from build123d import *

# Parameters (mm, degrees)
EXTRUDE_START       = -2
EXTRUDE_1_DEPTH     = 2
SKETCH_2_R          = 0.6
SKETCH_2_R_2        = 1.25
EXTRUDE_2_DEPTH     = 2
SKETCH_3_R          = 5.9
SKETCH_3_R_2        = 1.25
EXTRUDE_3_DEPTH     = 18.5
EXTRUDE_4_DEPTH     = 3
SKETCH_5_R          = 1.7
CUT_EXTRUDE_1_DEPTH = 3
SKETCH_6_R          = 1.7
EXTRUDE_5_DEPTH     = 4


# Read off the part's stored shape, not the designer's step: 填料-伸長1
with BuildPart() as part:
    # 填料-伸長1 outline → 填料-伸長1 (new body)
    with BuildSketch(Plane(origin=(0, 18.156954032, 0), x_dir=(1, 0, 0), z_dir=(0, 1, 0)).offset(EXTRUDE_START)):
        with BuildLine():
            Line((-71.976510321, -204.833021781), (-61.351692907, -213.569524655))
            ThreePointArc((-61.351692907, -213.569524655), (-59.430720516, -215.948258819), (-56.577073779, -217.046080048))
            Line((-56.577073779, -217.046080048), (-45.000342303, -224.475246616))
            ThreePointArc((-45.000342303, -224.475246616), (-39.06215434, -223.480955011), (-39.939141491, -217.524312868))
            Line((-39.939141491, -217.524312868), (-50.563958905, -208.787809993))
            ThreePointArc((-50.563958905, -208.787809993), (-52.484931295, -206.409075829), (-55.338578032, -205.311254601))
            Line((-55.338578032, -205.311254601), (-66.915309509, -197.882088033))
            ThreePointArc((-66.915309509, -197.882088033), (-72.853497472, -198.876379638), (-71.976510321, -204.833021781))
        make_face()
        with BuildLine():
            ThreePointArc((-55.939819286, -215.078625755), (-58.253468106, -214.331448143), (-59.674933886, -212.358967399))
            Line((-59.674933886, -212.358967399), (-70.741141252, -203.259521387))
            ThreePointArc((-70.741141252, -203.259521387), (-71.236686796, -200.053632048), (-68.033499603, -199.540910248))
            Line((-68.033499603, -199.540910248), (-55.975832526, -207.278708894))
            ThreePointArc((-55.975832526, -207.278708894), (-53.662183706, -208.025886506), (-52.240717926, -209.998367249))
            Line((-52.240717926, -209.998367249), (-41.17451056, -219.097813262))
            ThreePointArc((-41.17451056, -219.097813262), (-40.678965016, -222.303702601), (-43.882152209, -222.8164244))
            Line((-43.882152209, -222.8164244), (-55.939819286, -215.078625755))
        make_face(mode=Mode.SUBTRACT)
    extrude(amount=EXTRUDE_1_DEPTH)

    # 草圖2 → 填料-伸長2 (add)
    with BuildSketch(Plane(origin=(0, 18.156954032, 0), x_dir=(1, 0, 0), z_dir=(0, 1, 0))):
        with BuildLine():
            Line((-56.577073779, -217.046080048), (-45.000342303, -224.475246616))
            ThreePointArc((-45.000342303, -224.475246616), (-39.06215434, -223.480955011), (-39.939141491, -217.524312868))
            Line((-39.939141491, -217.524312868), (-50.563958905, -208.787809993))
            ThreePointArc((-50.563958905, -208.787809993), (-52.484931296, -206.409075829), (-55.338578032, -205.311254601))
            Line((-55.338578032, -205.311254601), (-66.915309509, -197.882088033))
            ThreePointArc((-66.915309509, -197.882088033), (-72.853497472, -198.876379638), (-71.976510321, -204.833021781))
            Line((-71.976510321, -204.833021781), (-61.351692907, -213.569524655))
            ThreePointArc((-61.351692907, -213.569524655), (-59.430720516, -215.948258819), (-56.577073779, -217.046080048))
        make_face()
        with Locations(Location((-69.943238255, -200.995433976, 0), (0, 0, 180))):
            Circle(SKETCH_2_R, mode=Mode.SUBTRACT)
        with Locations(Location((-68.245587045, -202.231549007, 0), (0, 0, 180))):
            Circle(SKETCH_2_R, mode=Mode.SUBTRACT)
        with Locations(Location((-66.547935835, -203.467664037, 0), (0, 0, 180))):
            Circle(SKETCH_2_R, mode=Mode.SUBTRACT)
        with Locations(Location((-64.850284625, -204.703779068, 0), (0, 0, 180))):
            Circle(SKETCH_2_R, mode=Mode.SUBTRACT)
        with Locations(Location((-63.152633415, -205.939894099, 0), (0, 0, 180))):
            Circle(SKETCH_2_R, mode=Mode.SUBTRACT)
        with Locations(Location((-61.454982205, -207.17600913, 0), (0, 0, 180))):
            Circle(SKETCH_2_R, mode=Mode.SUBTRACT)
        with Locations(Location((-55.957825906, -211.178667324, 0), (0, 0, 180))):
            Circle(SKETCH_2_R_2, mode=Mode.SUBTRACT)
        with Locations(Location((-50.460669607, -215.181325519, 0), (0, 0, 180))):
            Circle(SKETCH_2_R, mode=Mode.SUBTRACT)
        with Locations(Location((-48.763018397, -216.41744055, 0), (0, 0, 180))):
            Circle(SKETCH_2_R, mode=Mode.SUBTRACT)
        with Locations(Location((-47.065367187, -217.65355558, 0), (0, 0, 180))):
            Circle(SKETCH_2_R, mode=Mode.SUBTRACT)
        with Locations(Location((-45.367715977, -218.889670611, 0), (0, 0, 180))):
            Circle(SKETCH_2_R, mode=Mode.SUBTRACT)
        with Locations(Location((-43.670064767, -220.125785642, 0), (0, 0, 180))):
            Circle(SKETCH_2_R, mode=Mode.SUBTRACT)
        with Locations(Location((-41.972413557, -221.361900673, 0), (0, 0, 180))):
            Circle(SKETCH_2_R, mode=Mode.SUBTRACT)
    extrude(amount=EXTRUDE_2_DEPTH)

    # 草圖3 → 填料-伸長3 (add)
    with BuildSketch(Plane(origin=(0, 20.156954032, 0), x_dir=(1, 0, 0), z_dir=(0, 1, 0))):
        with Locations(Location((-55.957825906, -211.178667324, 0), (0, 0, 180))):
            Circle(SKETCH_3_R)
        with Locations(Location((-55.957825906, -211.178667324, 0), (0, 0, 180))):
            Circle(SKETCH_3_R_2, mode=Mode.SUBTRACT)
    extrude(amount=EXTRUDE_3_DEPTH)

    # 草圖4 → 填料-伸長4 (add)
    with BuildSketch(Plane(origin=(0, 38.656954032, 0), x_dir=(1, 0, 0), z_dir=(0, 1, 0))):
        Polygon((-59.623386181, -215.801833758), (-58.127150876, -205.691953447), (-122.426781037, -196.175779785), (-123.923016342, -206.285660097), align=None)
    extrude(amount=-EXTRUDE_4_DEPTH)

    # 草圖5 → 除料-伸長1 (cut)
    with BuildSketch(Plane.XZ.offset(-35.656954032)):
        with Locations((-65.8500767, 209.714640607)):
            Circle(SKETCH_5_R)
    extrude(amount=-CUT_EXTRUDE_1_DEPTH, mode=Mode.SUBTRACT)

    # 草圖6 → 填料-伸長5 (add)
    with BuildSketch(Plane(origin=(0, 28, 0), x_dir=(1, 0, 0), z_dir=(0, 1, 0))):
        with BuildLine():
            Line((-70.340889788, -205.906137252), (-71.251514406, -212.059117246))
            ThreePointArc((-71.251514406, -212.059117246), (-70.879084415, -213.543853469), (-69.565869591, -214.330372748))
            Line((-69.565869591, -214.330372748), (-59.623386181, -215.801833758))
            ThreePointArc((-59.623386181, -215.801833758), (-61.794253874, -210.314891561), (-58.127150876, -205.691953447))
            Line((-58.127150876, -205.691953447), (-68.069634286, -204.220492436))
            ThreePointArc((-68.069634286, -204.220492436), (-69.554370509, -204.592922428), (-70.340889788, -205.906137252))
        make_face()
        with Locations((-65.8500767, -209.714640607)):
            Circle(SKETCH_6_R, mode=Mode.SUBTRACT)
    extrude(amount=EXTRUDE_5_DEPTH)


solid = part.part
Read the model definition and answer for the solid it produces. Units are mm, in the model's axes. A direction names the side the tool comes from. Give positions to 0.01 mm unless a question says otherwise; leave off trailing zeros. Write each loop counter-clockwise with the first axis right and the second up, starting at its lowest first coordinate (ties: lowest second). Pieces come first, ordered by that corner, then holes. Notation, with made-up numbers: M 71,18.25 L 82,18.25 A27 cw 82,51.25 Z; hole C -6,-0.75 d8. An arc over 180 degrees is marked long. One line per item, written item: value. Start each with the question number.
(1) Find section B-B (x = -117.5). Determine the outline of the cut face in (y, z), plus the area to 3 significant figures.
(2) Flat-ended cylindrical pins translate along their axes: pin 1 Ø12 at (y, z) = (31, 210.5) entering from +X; pin 2 Ø1 at (x, z) = (-45.37, 218.89) entering from -Y; pin 3 Ø12 at (x, y) = (-86.5, 33) entering from +Z; pin 4 Ø6 at (x, z) = (-98, 203.5) entering from -Y. Find the tip coordinate at first contact, or state that the pin passes through.
(3) Determine the mould class of faces 4 (the flat face through (-68, 32, 210)), 5 (the cylindrical face through (-69.54, 29.97, 204.58)), 6 (the cylindrical face through (-56.63, 28.263, 212.233)), 7 (the flat face through (-56, 16.157, 207)) for opening direction Y: pulls with the +Y half, pulls with the -Y half, needs draft (parallel to the pull), parting line crosses it, or undercut.
(4) Find section C-C (y = 22). Determine the outline of the cut face in (x, z), plus the area to 3 significant figures.
(5) Find section A-A (y = 30.25). Determine the outline of the cut face in (x, z).
(6) Find the intervals of material crossed by line 1 (Y direction, x = -106.5, z = 201.5); line 2 (Y direction, x = -52.5, z = 218.25); line 3 (X direction, y = 19.75, z = 218.75), in increasing order.
(7) A tool of negligible diameter and unlimited length cuts with its end or side. For faces 1 (the flat face through (-123.164, 37.178, 201.16)), 2 (the cylindrical face through (-66.219, 37.136, 208.055)), 3 (the cylindrical face through (-53.7, 17.1, 208)), from which of +Z, -Z, +X, -X, +Y, -Y can it reach the whole face along a straight path? Write none if from no direction.
Results below:
1. outline: M 35.66,196.9 L 38.66,196.9 L 38.66,207.24 L 35.66,207.24 Z
1. area: 31.0 mm^2
2. pin 1: stops at x = -50.06
2. pin 2: passes through
2. pin 3: stops at z = 212.62
2. pin 4: stops at y = 35.66
3. face 4: undercut
3. face 5: undercut
3. face 6: needs draft
3. face 7: pulls with the -Y half
4. outline: C -55.96,211.18 d11.8; hole C -55.96,211.18 d2.5
4. area: 104 mm^2
5. outline: M -71.25,212.06 L -70.34,205.91 A2 ccw -68.07,204.22 L -58.13,205.69 A5.9 ccw long -59.62,215.8 L -69.57,214.33 A2 ccw Z; hole C -65.85,209.71 d3.4; hole C -55.96,211.18 d2.5
6. line 1: y = 35.66 to 38.66
6. line 2: y = 16.16 to 20.16
6. line 3: x = -53.92 to -45.95, -44.78 to -38.84
7. face 1: -Z, -X, +Y, -Y
7. face 2: +Y
7. face 3: -Y
